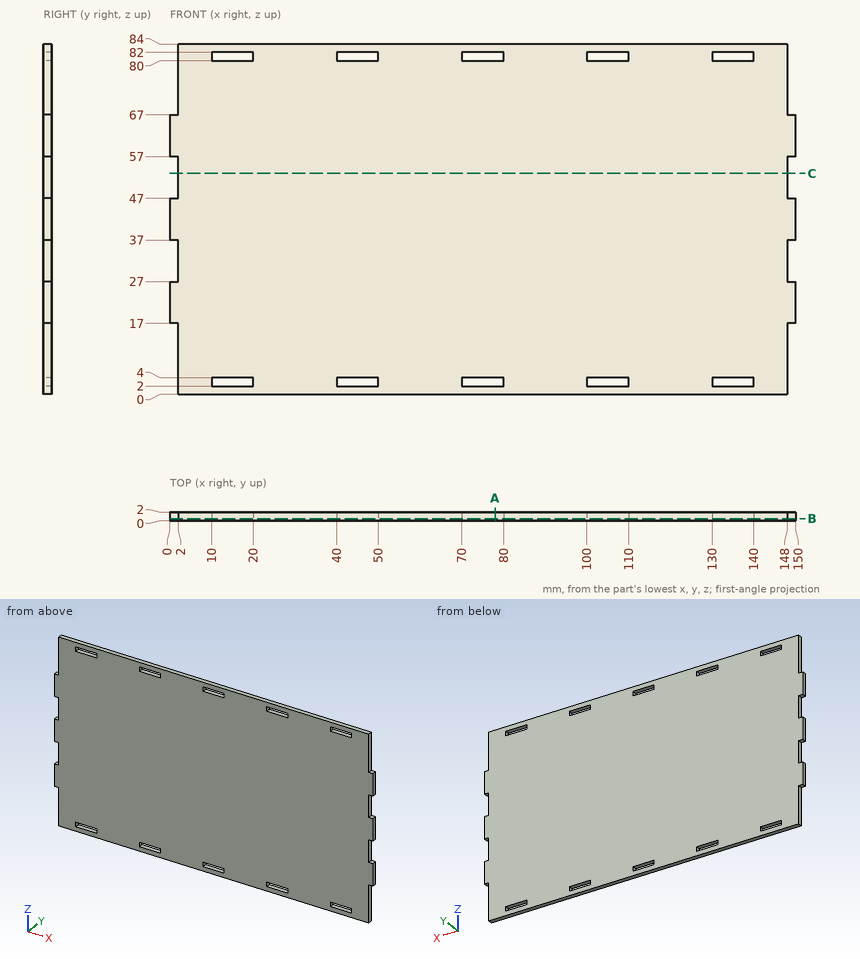
Study the drawing (mm; zero at the part's minimum x, y, z) and answer. Give positions to 0.01 mm unless a question says otherwise; leave off trailing zeros. Loops run counter-clockwise (first coordinate to the right, second up) from the corner with the lowest first, then second, coordinate; pieces in that order, holes last. Notation, with made-up numbers: (-8, 69) -> (43, 69) arc R31 ccw to (43, 97) -> close; hole circle Ø6 at (-16.5, -10.5). An arc over 180 degrees is marked (long way). Write item = value, one per line. Start each with the question number.
(1) Find section B-B on y = 0.5. Give the number of separate pieces and of enclosed holes in the cut face, and give its area (3 significant figures).
(2) Find section C-C on z = 53. Give the vertices of the cut face in (x, y).
(3) Find the intervals of material crossed by probe 1 along Z at (x, y) = (138, 1.05); probe 2 along X at (y, z) = (1.85, 31), in increasing order. Write a range as from..to.
(4) Given pin 1 Ø1 at (y, z) = (1.5, 3) entering from +X; pin 2 Ø1 at (x, y) = (149, 1) entering from -Z; pin 3 Ø0.6 at (y, z) = (1, 81) entering from -X, each flat-ended and moving along its own axis, determine where each tip first touches the part or whether it passes through.
(5) Find section A-A on x = 78. Give the vertices of the cut face in (y, z), and give its area (3 significant figures).
From the geometry:
q1.separate_pieces = 1
q1.enclosed_holes = 10
q1.area = 12,200 mm^2
q2.outline = (2, 0) -> (148, 0) -> (148, 2) -> (2, 2) -> close
q3.probe_1 = 0..2, 4..80, 82..84
q3.probe_2 = 2..148
q4.pin_1 = 148
q4.pin_2 = 17
q4.pin_3 = 2
q5.outline = (0, 0) -> (2, 0) -> (2, 2) -> (0, 2) -> close; (0, 4) -> (2, 4) -> (2, 80) -> (0, 80) -> close; (0, 82) -> (2, 82) -> (2, 84) -> (0, 84) -> close
q5.area = 160 mm^2
